Here's how the part is built. I have some questions about the finished solid (model axes, mm). Face numbers are marked on the shaded views. A direction names the side the tool comes from. Coordinates: 2 decimals unless noted, no trailing zeros. Loops run counter-clockwise (first coordinate to the right, second up) from the corner with the lowest first, then second, coordinate; pieces in that order, holes last. Notation, with made-up numbers: M 8.25,-17 L 49.25,-17 A20 ccw 49.25,15 Z; hole C 61.25,26 d9. An arc over 180 degrees is marked long. Use one line per item in the form item = value. Start each with the question number.
(1) Imagine slicing it at C-C, the plane z = 30. Please give me the cut outline in (x, y), and give its area (3 significant figures).
(2) Will these pins go through, and if not, where does the flat tip stop? P1, Ø5.5, axis at x = -24.5, y = 38.5, coming from the +Z side; P2, Ø2, axis at x = -42, y = 35, coming from the -Z side; P3, Ø6, axis at x = -44.5, z = 40.5, coming from the -Y side; P4, Ø6.5, axis at y = 39.4, z = -4.32, coming from the -X side.
(3) On a 3-axis mill with a long thin cutter (end or side, diameter ignored), from which of +Z, -Z, +X, -X, +Y, -Y can I reach the whole of each face in a straight line? I mean the marked faces 1, 2, 3 and 4. Say none if no direction works.
(4) Imagine slicing it at B-B, the plane y = 30. Please give me the cut outline in (x, z), and give its area (3 significant figures).
(5) Please list where these lines run through material, in increasing order: L1, parallel to X at y = 43, z = 34; L2, parallel to Z at x = -21.5, y = 28.25.
(6) Imagine slicing it at D-D, the plane z = 21. Please give me the cut outline in (x, y).
(7) Imagine slicing it at A-A, the plane x = -15. Please give me the cut outline in (y, z), and give its area (3 significant figures).
```python
from build123d import *

# Parameters (mm, degrees)
SKETCH_1_W          = 37.5
SKETCH_1_H          = 19.5
EXTRUDE_1_DEPTH     = 40
SKETCH_2_W          = 7
SKETCH_2_H          = 19.5
EXTRUDE_2_DEPTH     = 3
CUT_EXTRUDE_START   = -70.872542033
SKETCH_3_R          = 2
CUT_EXTRUDE_5_DEPTH = 73.872542033
SKETCH_4_R          = 2.45
EXTRUDE_3_DEPTH     = 4
FILLET_1_R          = 0.5


with BuildPart() as part:
    # Sketch 1 → Extrude 1 (new body)
    with BuildSketch(Plane.XY):
        with Locations((-27.096153846, 34.403846154)):
            Rectangle(SKETCH_1_W, SKETCH_1_H)
    extrude(amount=EXTRUDE_1_DEPTH)

    # Sketch 2 → Extrude 2 (add)
    with BuildSketch(Plane.ZY.offset(35.246153846)):
        with Locations((-3.5, 34.403846154)):
            Rectangle(SKETCH_2_W, SKETCH_2_H)
        with Locations((43.5, 34.403846154)):
            Rectangle(SKETCH_2_W, SKETCH_2_H)
    extrude(amount=EXTRUDE_2_DEPTH)

    # Sketch 3 → Cut-Extrude 5 (cut)
    with BuildSketch(Plane.ZY.offset(35.246153846).offset(CUT_EXTRUDE_START)):
        with Locations(Location((-4.315, 39.403846154, 0), (0, 0, 90))):
            Circle(SKETCH_3_R)
        with Locations(Location((-4.315, 29.403846154, 0), (0, 0, 90))):
            Circle(SKETCH_3_R)
    cut_extrude_5 = extrude(amount=CUT_EXTRUDE_5_DEPTH, mode=Mode.SUBTRACT)

    # Sketch 4 → Extrude 3 (add)
    with BuildSketch(Plane.ZY.offset(45.846153846)):
        with Locations(Location((30, 34.403846154, 0), (0, 0, 90))):
            Circle(SKETCH_4_R)
    extrude(amount=EXTRUDE_3_DEPTH)

    # Fillet 1
    fillet_1_edges = [part.edges().sort_by_distance(p)[0] for p in [
        (-42.046153846, 44.153846154, 40),
        (-21.796153846, 44.153846154, 0),
        (-21.796153846, 24.653846154, 0),
        (-35.246153846, 34.403846154, 0),
        (-35.246153846, 44.153846154, -3.5),
        (-36.746153846, 44.153846154, -7),
        (-35.246153846, 24.653846154, -3.5),
        (-36.746153846, 24.653846154, -7),
        (-38.246153846, 34.403846154, 0),
        (-38.246153846, 44.153846154, -3.5),
        (-38.246153846, 24.653846154, -3.5),
        (-21.796153846, 24.653846154, 40),
        (-21.796153846, 44.153846154, 40),
        (-35.246153846, 34.403846154, 40),
        (-35.246153846, 24.653846154, 43.5),
        (-36.746153846, 24.653846154, 47),
        (-35.246153846, 44.153846154, 43.5),
        (-36.746153846, 44.153846154, 47),
        (-38.246153846, 34.403846154, 40),
        (-38.246153846, 24.653846154, 43.5),
        (-38.246153846, 44.153846154, 43.5),
        (-42.046153846, 44.153846154, 0),
        (-49.846153846, 31.953846154, 30),
        (-42.046153846, 24.653846154, 0),
        (-42.046153846, 24.653846154, 40),
    ]]
    fillet(fillet_1_edges, radius=FILLET_1_R)

    # Mirror 1: Cut-Extrude 5 across plane
    add(cut_extrude_5.mirror(Plane(origin=(0, 0, 20), x_dir=(1, 0, 0), z_dir=(0, 0, -1))), mode=Mode.SUBTRACT)


solid = part.part
```
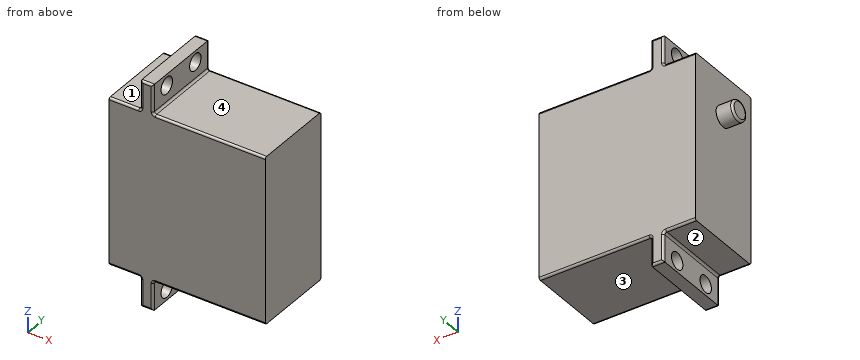
Answer:
q1.outline = M -49.85,32.45 A0.5 ccw -49.35,31.95 L -45.85,31.95 L -45.85,24.65 L -8.35,24.65 L -8.35,44.15 L -45.85,44.15 L -45.85,36.85 L -49.35,36.85 A0.5 ccw -49.85,36.35 Z
q1.area = 751 mm²
q2.P1 = 40
q2.P2 = 0
q2.P3 = 24.65
q2.P4 = -38.25
q3.face_1 = +Z, -X, +Y, -Y
q3.face_2 = -Z, -X, +Y, -Y
q3.face_3 = -Z, +X, +Y, -Y
q3.face_4 = +Z, +X, +Y, -Y
q4.outline = M -45.85,0 L -38.75,0 A0.5 cw -38.25,-0.5 L -38.25,-2.41 L -35.25,-2.41 L -35.25,-0.5 A0.5 cw -34.75,0 L -8.35,0 L -8.35,40 L -34.75,40 A0.5 cw -35.25,40.5 L -35.25,42.41 L -38.25,42.41 L -38.25,40.5 A0.5 cw -38.75,40 L -45.85,40 Z; M -38.25,-7 L -35.25,-7 L -35.25,-6.22 L -38.25,-6.22 Z; M -38.25,46.22 L -35.25,46.22 L -35.25,47 L -38.25,47 Z
q4.area = 1,520 mm²
q5.L1 = -45.85 to -8.35
q5.L2 = 0 to 40
q6.outline = M -45.85,24.65 L -8.35,24.65 L -8.35,44.15 L -45.85,44.15 Z
q7.outline = M 24.65,0.5 A0.5 ccw 25.15,0 L 43.65,0 A0.5 ccw 44.15,0.5 L 44.15,39.5 A0.5 ccw 43.65,40 L 25.15,40 A0.5 ccw 24.65,39.5 Z
q7.area = 780 mm²
